from build123d import *

# Parameters (mm, degrees)
CROQUIS1_R              = 10
SALIENTE_EXTRUIR1_DEPTH = 8
CROQUIS2_R              = 5
SALIENTE_EXTRUIR2_DEPTH = 20
CHAFL_N1_SIZE           = 1
CHAFL_N2_SIZE           = 1


with BuildPart() as part:
    # Croquis1 → Saliente-Extruir1 (new body)
    with BuildSketch(Plane.XY):
        Circle(CROQUIS1_R)
    extrude(amount=SALIENTE_EXTRUIR1_DEPTH)

    # Croquis2 → Saliente-Extruir2 (add)
    with BuildSketch(Plane.XY.offset(8)):
        Circle(CROQUIS2_R)
    extrude(amount=SALIENTE_EXTRUIR2_DEPTH)

    # Chaflán1
    chafl_n1_edges = [part.edges().sort_by_distance(p)[0] for p in [
        (-10, 0, 0),
        (-10, 0, 8),
    ]]
    chamfer(chafl_n1_edges, length=CHAFL_N1_SIZE)

    # Chaflán2
    chafl_n2_edges = [part.edges().sort_by_distance(p)[0] for p in [
        (-5, 0, 28),
    ]]
    chamfer(chafl_n2_edges, length=CHAFL_N2_SIZE)


solid = part.part
For this review, take the finished solid that the model builds, in its own axes (mm). A direction names the side the tool comes from. Round coordinates to 2 decimals unless told otherwise and drop trailing zeros. Write each loop counter-clockwise with the first axis right and the second up, starting at its lowest first coordinate (ties: lowest second). Pieces come first, ordered by that corner, then holes. Notation, with made-up numbers: (72.5, -22) -> (98.5, -22) arc R19 cw to (98.5, -12) -> close; hole circle Ø8 at (60, 56). An arc over 180 degrees is marked (long way). Use CSV: the item, a comma, the result in double quotes.
(1) For faces 1 (the face through (-1.08, -4.88, 17.37)), 2 (the face through (0, 0, 28)), list the 3-axis set-ups (+Z, -Z, +X, -X, +Y, -Y) from which the entire face can be reached by the end or side of a thin tool; tool diameter is ignored.
Computed values:
face 1,"+Z"
face 2,"+Z, +X, -X, +Y, -Y"
(2) Clearance check with flat-ended pins moving along their axes: P1, Ø12, axis at x = 7.5, z = 23.5, coming from the -Y side; P2, Ø12, axis at x = -4, y = -6.5, coming from the -Z side; P3, Ø4, axis at y = 6, z = 12, coming from the +X side; P4, Ø3, axis at y = 5, z = 12, coming from the +X side. State where each tip first meets the part, or that it passes through.
Computed values:
P1,"y = -4.77"
P2,"z = 0"
P3,"x = 3"
P4,"x = 3.57"
(3) Consider section A-A, the plane y = 0. Give the boundary of the cut face in (x, z).
Computed values:
outline,"(-10, 1) -> (-9, 0) -> (9, 0) -> (10, 1) -> (10, 7) -> (9, 8) -> (5, 8) -> (5, 27) -> (4, 28) -> (-4, 28) -> (-5, 27) -> (-5, 8) -> (-9, 8) -> (-10, 7) -> close"
(4) Consider section C-C, the plane z = 21. Give the boundary of the cut face in (x, y), plus the area to 3 significant figures.
Computed values:
outline,"circle Ø10 at (0, 0)"
area,"78.5 mm²"
(5) To check wall thickness, follow L1, parallel to Y at x = 0, z = 21; L2, parallel to Z at x = -8.5, y = 2.25; L3, parallel to X at y = 3, z = 24. State the ranges of each line that lie inside material, in increasing order. Write a range as [from, to].
Computed values:
L1,"[-5, 5]"
L2,"[0, 8]"
L3,"[-4, 4]"
(6) Consider section D-D, the plane z = 6. Give the boundary of the cut face in (x, y).
Computed values:
outline,"circle Ø20 at (0, 0)"
